Here's how the part is built. I have some questions about the finished solid (model axes, mm). Give positions to 0.01 mm unless a question says otherwise; leave off trailing zeros. Loops run counter-clockwise (first coordinate to the right, second up) from the corner with the lowest first, then second, coordinate; pieces in that order, holes last. Notation, with made-up numbers: (-22.5, 75.25) - (-7.5, 75.25) arc R17 ccw to (-7.5, 99.25) - close; hole circle Ø11 at (62, 83). An arc over 180 degrees is marked (long way). One line per item, written item: value. Start each with the question number.
Autodesk Inventor part; units mm, degrees
ref_plane "YZ Plane" through (0, 0, 0) normal (1, 0, 0) x (0, 1, 0)
ref_plane "XZ Plane" through (0, 0, 0) normal (0, 1, 0) x (-1, 0, 0)
ref_plane "XY Plane" through (0, 0, 0) normal (0, 0, 1) x (1, 0, 0)
sketch "Sketch1" plane through (0, 0, 0) normal (0, 0, 1) x (1, 0, 0)
  circle A0 centre (21, 0) radius 2.25
  circle A1 centre (-21, 0) radius 2.25
  line L0 (21, 0) -> (-21, 0) construction
  line L1 (21, 4) -> (-21, 4)
  line L2 (-21, -4) -> (21, -4)
  arc A2 (21, -4) -> (21, 4) centre (21, 0) ccw
  arc A3 (-21, 4) -> (-21, -4) centre (-21, 0) ccw
  point P0 (0, 0)
  point P1 (0, 0)
  dimension "d0" = 8
extrude "Extrusion1" add sketch "Sketch1" along normal blind 6
scale "Scale1" factors (0.5, 0.5, 0.5) then translate (0, -2, 3) bodies 1
properties part number "MassiveToe2"
(1) If we section it at D-D on y = -3.7: List the corners of the cut face in (x, z) for me.
(2) Please list where these lines run through material, in increasing order: probe 1 along X at (y, z) = (-2.05, 4.5); probe 2 along Y at (x, z) = (10.5, 4.95) (3 decimals); probe 3 along X at (y, z) = (-2.55, 4.2). Write a range as from..to.
(3) If we mould it in two halves opening along Y, with no side actions, what happens to faces 1 (the face through (-12.5, -2, 4.5)), 2 (the face through (11.573, -2.338, 4.479)), 3 (the face through (0, 0, 4))? For each: pulls with the +Y half, pulls with the -Y half, needs draft (parallel to the pull), parting line crosses it, or undercut.
(4) If we section it at C-C on x = 11.25: List the corners of the cut face in (y, z) for me.
(5) If we section it at A-A on y = -2: List the corners of the cut face in (x, z) for me (3 decimals), plus the area to 3 significant figures.
(6) If we section it at B-B on z = 4.2: List the corners of the cut face in (x, y) for me (3 decimals).
Found:
1. outline: (-11.55, 3) - (11.55, 3) - (11.55, 6) - (-11.55, 6) - close
2. probe 1: -12.5..-11.62, -9.38..9.38, 11.62..12.5
2. probe 2: -4..-3.125, -0.875..0
2. probe 3: -12.42..-11.48, -9.52..9.52, 11.48..12.42
3. face 1: parting line crosses it
3. face 2: undercut
3. face 3: pulls with the +Y half
4. outline: (-3.85, 3) - (-2.84, 3) - (-2.84, 6) - (-3.85, 6) - close; (-1.16, 3) - (-0.15, 3) - (-0.15, 6) - (-1.16, 6) - close
5. outline: (-12.5, 3) - (-11.625, 3) - (-11.625, 6) - (-12.5, 6) - close; (-9.375, 3) - (9.375, 3) - (9.375, 6) - (-9.375, 6) - close; (11.625, 3) - (12.5, 3) - (12.5, 6) - (11.625, 6) - close
5. area: 61.5 mm^2
6. outline: (-10.5, -4) - (10.5, -4) arc R2 ccw to (10.5, 0) - (-10.5, 0) arc R2 ccw to start; hole circle Ø2.25 at (-10.5, -2); hole circle Ø2.25 at (10.5, -2)
